Verification items for this drawing (mm, ordinates from the low corner). A direction names the side the tool comes from. Coordinates: 2 decimals unless noted, no trailing zeros. Order: outer loops, then holes, each group sorted by start corner. A loop starts at its lowest first (then second) coordinate and runs counter-clockwise, first axis right, second up. Notation, with made-up numbers: M 79,-36 L 88,-36 A21 cw 88,-2 Z; hole C 0,-36.5 d10. An arc over 180 degrees is marked long. Return JSON: item names as keys, results as strings. Group by question number.
1. Gauge pin test, flat ends, axial feed: pin 1 (8 mm diameter, centred on y = 25.5, z = 11.5, fed in from +X); pin 2 (1 mm diameter, centred on y = 25, z = 20, fed in from -X); pin 3 (3 mm diameter, centred on x = 11, y = 13, fed in from +Z); pin 4 (10 mm diameter, centred on x = 22, y = 25, fed in from -Z). Record the tip position at first contact, or that the pin passes through.
2. Section check A-A, the plane x = 20. Record the cut outline in (y, z), plus the area to 3 significant figures.
3. Material ranges on line 1 along Z through (x, y) = (11, 9); line 2 along Z through (x, y) = (15, 21); line 3 along Y through (x, z) = (33, 16.5), recorded low to high.
4. Set-up check for the marked faces 1 and 2: record each of +Z, -Z, +X, -X, +Y, -Y from which the full face is reachable in a straight line by a thin tool's end or side.
5. Section check D-D, the plane z = 9.5. Record the cut outline in (x, y), plus the area to 3 significant figures.
6. Section check C-C, the plane z = 44. Record the cut outline in (x, y), plus the area to 3 significant figures.
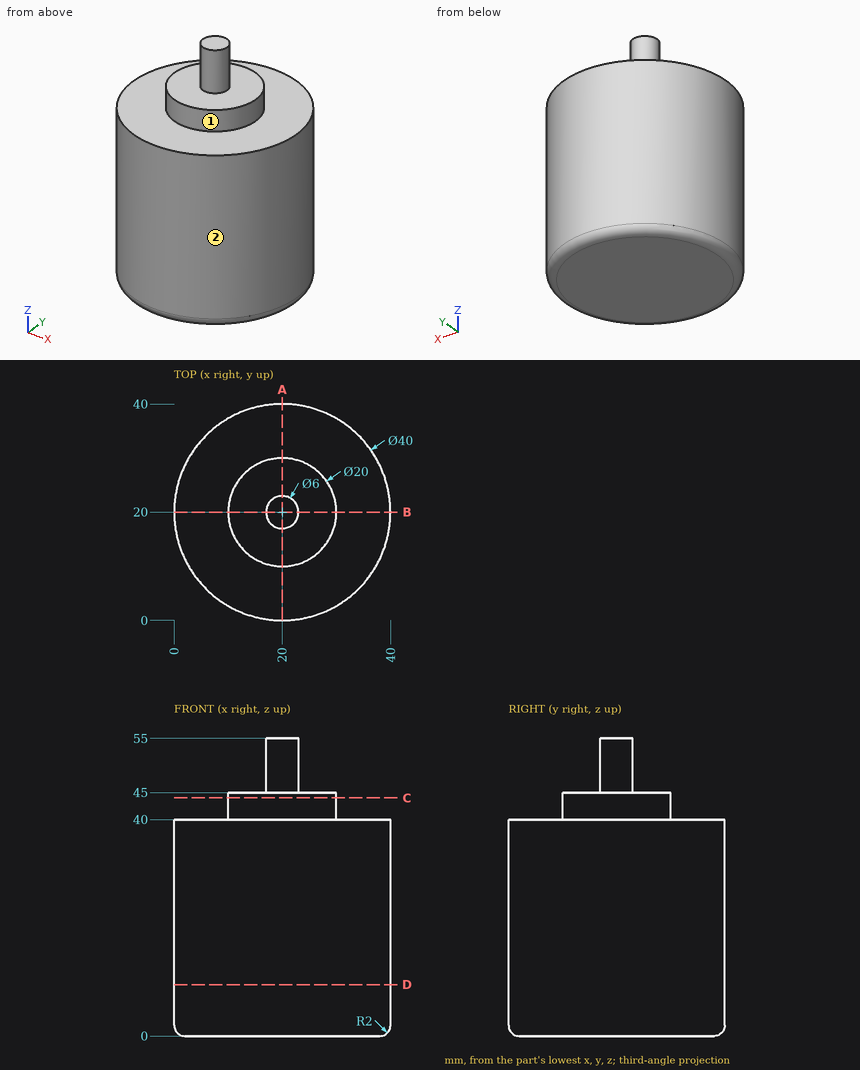
Answers follow:
{
 "1": {"pin 1": "x = 39.94", "pin 2": "x = 0.51", "pin 3": "z = 45", "pin 4": "z = 0"},
 "2": {"outline": "M 0,2 A2 ccw 2,0 L 38,0 A2 ccw 40,2 L 40,40 L 30,40 L 30,45 L 23,45 L 23,55 L 17,55 L 17,45 L 10,45 L 10,40 L 0,40 Z", "area": "1,760 mm^2"},
 "3": {"line 1": "0 to 40", "line 2": "0 to 45", "line 3": "4.8 to 35.2"},
 "4": {"face 1": "+Z", "face 2": "+Z, -Z"},
 "5": {"outline": "C 20,20 d40", "area": "1,260 mm^2"},
 "6": {"outline": "C 20,20 d20", "area": "314 mm^2"}
}
